Autodesk Inventor part; units mm, degrees
ref_plane "YZ Plane" through (0, 0, 0) normal (1, 0, 0) x (0, 1, 0)
ref_plane "XZ Plane" through (0, 0, 0) normal (0, 1, 0) x (-1, 0, 0)
ref_plane "XY Plane" through (0, 0, 0) normal (0, 0, 1) x (1, 0, 0)
sketch "Sketch1" plane through (0, 0, 0) normal (0, 1, 0) x (-1, 0, 0)
  line L0 (0.9108, 1.27) -> (-0.9108, 1.27)
  line L1 (-0.9108, 1.27) -> (-1.27, 0.9108)
  line L2 (-1.27, 0.9108) -> (-1.27, -0.9108)
  line L3 (0.9108, -1.27) -> (1.27, -0.9108)
  line L4 (1.27, -0.9108) -> (1.27, 0.9108)
  line L5 (0.9108, 1.27) -> (1.27, 0.9108)
  line L6 (-1.27, -0.9108) -> (-0.9108, -1.27)
  line L7 (-0.9108, -1.27) -> (0.9108, -1.27)
  line L8 (-1.27, 0) -> (1.27, 0) construction
  point P0 (0, 0)
  point P1 (0, 0)
  dimension "d1" = 2.54
  dimension "d3" = 0.508
  dimension "d4" = 135
extrude "Extrusion1" add sketch "Sketch1" along normal blind 2.54
sketch "Sketch2" plane through (0, 2.54, 0) normal (0, 1, 0) x (1, 0, 0)
  line L0 (-0.3175, 0.3175) -> (0.3175, 0.3175)
  line L1 (0.3175, 0.3175) -> (0.3175, -0.3175)
  line L2 (0.3175, -0.3175) -> (-0.3175, -0.3175)
  line L3 (-0.3175, -0.3175) -> (-0.3175, 0.3175)
  line L4 (-0.3175, 0.3175) -> (0.3175, -0.3175) construction
  point P0 (0, 0)
  point P1 (0, 0)
  dimension "d7" = 0.635
extrude "Extrusion2" add sketch "Sketch2" along normal blind 5.08
properties part number "Header1x1"
Verification items for the finished model (mm, model axes). Coordinates: 2 decimals unless noted, no trailing zeros. Write each loop counter-clockwise with the first axis right and the second up, starting at its lowest first coordinate (ties: lowest second). Pieces come first, ordered by that corner, then holes. Notation, with made-up numbers: (-31.75, 85.25) - (12.25, 85.25) arc R10 ccw to (12.25, 95.25) - close; hole circle Ø4 at (82.25, -31.75). An arc over 180 degrees is marked (long way). One line per question, with ' | ' between items. Start each with the question number.
1. Gauge pin test, flat ends, axial feed: P1, Ø1.5, axis at y = 6.5, z = 0.5, coming from the -X side; P2, Ø0.7, axis at x = 0, y = 4.5, coming from the +Z side; P3, Ø1.5, axis at x = 0, y = 4.5, coming from the -Z side. Record the tip position at first contact, or that the pin passes through.
2. Section check D-D (x = -0.5). Enter the section's corners in (y, z).
3. Section check B-B (y = 2). Enter the section's corners in (x, z).
4. Section check C-C (z = -0.7). Enter the section's corners in (x, y), plus the area to 3 significant figures.
5. Material ranges on line 1 along X through (y, z) = (4, 0.15); line 2 along Y through (x, z) = (0.85, -1.05), recorded low to high.
6. Section check A-A (x = -0.2). Enter the section's corners in (y, z), plus the area to 3 significant figures.
Computed values:
1) P1: x = -0.32 | P2: z = 0.32 | P3: z = -0.32
2) outline: (0, -1.27) - (2.54, -1.27) - (2.54, 1.27) - (0, 1.27) - close
3) outline: (-1.27, -0.91) - (-0.91, -1.27) - (0.91, -1.27) - (1.27, -0.91) - (1.27, 0.91) - (0.91, 1.27) - (-0.91, 1.27) - (-1.27, 0.91) - close
4) outline: (-1.27, 0) - (1.27, 0) - (1.27, 2.54) - (-1.27, 2.54) - close | area: 6.45 mm²
5) line 1: -0.32 to 0.32 | line 2: 0 to 2.54
6) outline: (0, -1.27) - (2.54, -1.27) - (2.54, -0.32) - (7.62, -0.32) - (7.62, 0.32) - (2.54, 0.32) - (2.54, 1.27) - (0, 1.27) - close | area: 9.68 mm²
